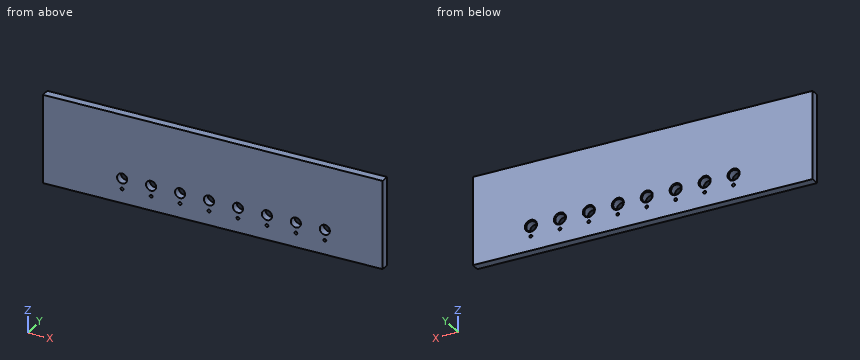
from build123d import *

# Parameters (mm, degrees)
ESQUISSE5_W             = 352
ESQUISSE5_H             = 93
BOSS_EXTRU_2_DEPTH      = 8.5
ESQUISSE3_R             = 1.5
ESQUISSE3_R_2           = 5.25
ENL_V_MAT_EXTRU_1_DEPTH = 9.5
CHANFREIN1_SIZE         = 1


with BuildPart() as part:
    # Esquisse5 → Boss.-Extru.2 (new body)
    with BuildSketch(Plane(origin=(0, 0, 0), x_dir=(1, 0, 0), z_dir=(0, 1, 0))):
        with Locations((5, -46.5)):
            Rectangle(ESQUISSE5_W, ESQUISSE5_H)
    extrude(amount=-BOSS_EXTRU_2_DEPTH)

    # Esquisse3 → Enlèv. mat.-Extru.1 (cut, through all)
    with BuildSketch(Plane(origin=(0, 0, 0), x_dir=(1, 0, 0), z_dir=(0, 1, 0))):
        with Locations((-89, -15)):
            Circle(ESQUISSE3_R)
        with Locations((-89, -26)):
            Circle(ESQUISSE3_R_2)
        with Locations((-59, -15)):
            Circle(ESQUISSE3_R)
        with Locations((-59, -26)):
            Circle(ESQUISSE3_R_2)
        with Locations((-29, -15)):
            Circle(ESQUISSE3_R)
        with Locations((-29, -26)):
            Circle(ESQUISSE3_R_2)
        with Locations((1, -15)):
            Circle(ESQUISSE3_R)
        with Locations((1, -26)):
            Circle(ESQUISSE3_R_2)
        with Locations((31, -15)):
            Circle(ESQUISSE3_R)
        with Locations((31, -26)):
            Circle(ESQUISSE3_R_2)
        with Locations((61, -15)):
            Circle(ESQUISSE3_R)
        with Locations((61, -26)):
            Circle(ESQUISSE3_R_2)
        with Locations((91, -15)):
            Circle(ESQUISSE3_R)
        with Locations((91, -26)):
            Circle(ESQUISSE3_R_2)
        with Locations((121, -15)):
            Circle(ESQUISSE3_R)
        with Locations((121, -26)):
            Circle(ESQUISSE3_R_2)
    extrude(amount=-ENL_V_MAT_EXTRU_1_DEPTH, mode=Mode.SUBTRACT)

    # Chanfrein1
    chanfrein1_edges = [part.edges().sort_by_distance(p)[0] for p in [
        (-34.25, 0, 26),
        (-4.25, 0, 26),
        (-94.25, 0, 26),
        (-64.25, 0, 26),
        (85.75, 0, 26),
        (115.75, 0, 26),
        (25.75, 0, 26),
        (55.75, 0, 26),
    ]]
    chamfer(chanfrein1_edges, length=CHANFREIN1_SIZE)


solid = part.part
Can you work these out from the model? Positions are in its coordinate system, mm. Give positions to 0.01 mm unless a question says otherwise; leave off trailing zeros. Answer in a Markdown table with one row per item. Add a question column.
Item 1: Imagine slicing it at A-A, the plane y = -6.5. State how many separate pieces and enclosed holes the cut face has, plus the area to 3 significant figures.
Item 2: Please list where these lines run through material, in increasing order: L1, parallel to Z at x = 1, y = -1.75; L2, parallel to Z at x = -32, y = -7.25.
Item 3: For pin 1 Ø2.5 at (x, z) = (91, 15) entering from +Y, with a flat end and sliding along its axis, tell me the tip position at first contact or that it passes through.
Evaluation:
| question | item | result |
|---|---|---|
| 1 | separate pieces | 1 |
| 1 | enclosed holes | 16 |
| 1 | area | 32,000 mm² |
| 2 | L1 | z = 0 to 13.5, 16.5 to 20.75, 31.25 to 93 |
| 2 | L2 | z = 0 to 21.69, 30.31 to 93 |
| 3 | pin 1 | passes through |
